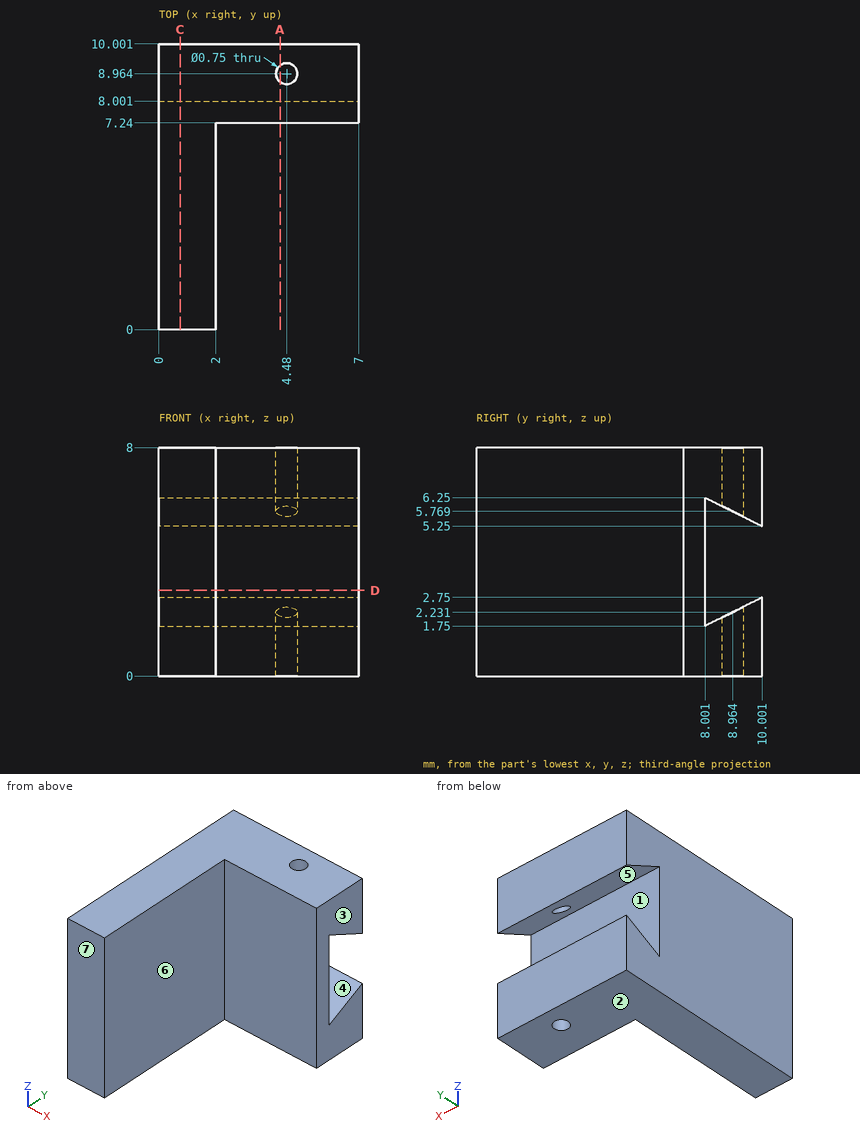
Geometry check sheet. Reference: drawing and pictorial views, mm from the part's lowest x, y, z. A direction names the side the tool comes from. Round coordinates to 2 decimals unless told otherwise and drop trailing zeros. Loops run counter-clockwise (first coordinate to the right, second up) from the corner with the lowest first, then second, coordinate; pieces in that order, holes last. Notation, with made-up numbers: (53.25, 33.25) - (88.25, 33.25) arc R20 cw to (88.25, 42.25) - close; hole circle Ø1 at (63, 78.5). An arc over 180 degrees is marked (long way). One line per question, with ' | ' between items. Start each with the question number.
1. Cross-section at C-C on x = 0.75. Record the cut outline in (y, z).
2. Cross-section at D-D on z = 3. Record the cut outline in (x, y).
3. Tool access check on the marked faces 5, 6 and 7. Record the directions out of +Z, -Z, +X, -X, +Y, -Y that give a thin tool (end or side, any length) a straight path to the whole face; none if there is none.
4. Scan lines: line 1 (Y direction, x = 5.25, z = 0.75); line 2 (Y direction, x = 0.5, z = 4.5); line 3 (Z direction, x = 1.5, y = 9). Record each from-to range of solid material in increasing order. Write a range as [from, to].
5. Draft check along Z on the marked faces 1, 2, 3 and 4. Enter one of: released by +Z, released by -Z, zero draft, split by the parting line, or undercut.
6. Depth check by flat-ended pin: pin 1 (1.5 mm diameter, centred on x = 4.5, z = 5.5, fed in from -Y). Enter the tip coordinate at first touch or a pass-through.
7. Cross-section at A-A on x = 4.25. Record the cut outline in (y, z).
Taken from the geometry:
1) outline: (0, 0) - (10, 0) - (10, 2.75) - (8, 1.75) - (8, 6.25) - (10, 5.25) - (10, 8) - (0, 8) - close
2) outline: (0, 0) - (2, 0) - (2, 7.24) - (7, 7.24) - (7, 8) - (0, 8) - close
3) face 5: +X, -X | face 6: +Z, -Z, +X, -Y | face 7: +Z, -Z, +X, -X, -Y
4) line 1: [7.24, 10] | line 2: [0, 8] | line 3: [0, 2.25], [5.75, 8]
5) face 1: undercut | face 2: released by -Z | face 3: zero draft | face 4: undercut
6) pin 1: y = 7.24
7) outline: (7.24, 0) - (8.67, 0) - (8.67, 2.08) - (8, 1.75) - (8, 6.25) - (8.67, 5.92) - (8.67, 8) - (7.24, 8) - close; (9.26, 0) - (10, 0) - (10, 2.75) - (9.26, 2.38) - close; (9.26, 5.62) - (10, 5.25) - (10, 8) - (9.26, 8) - close
